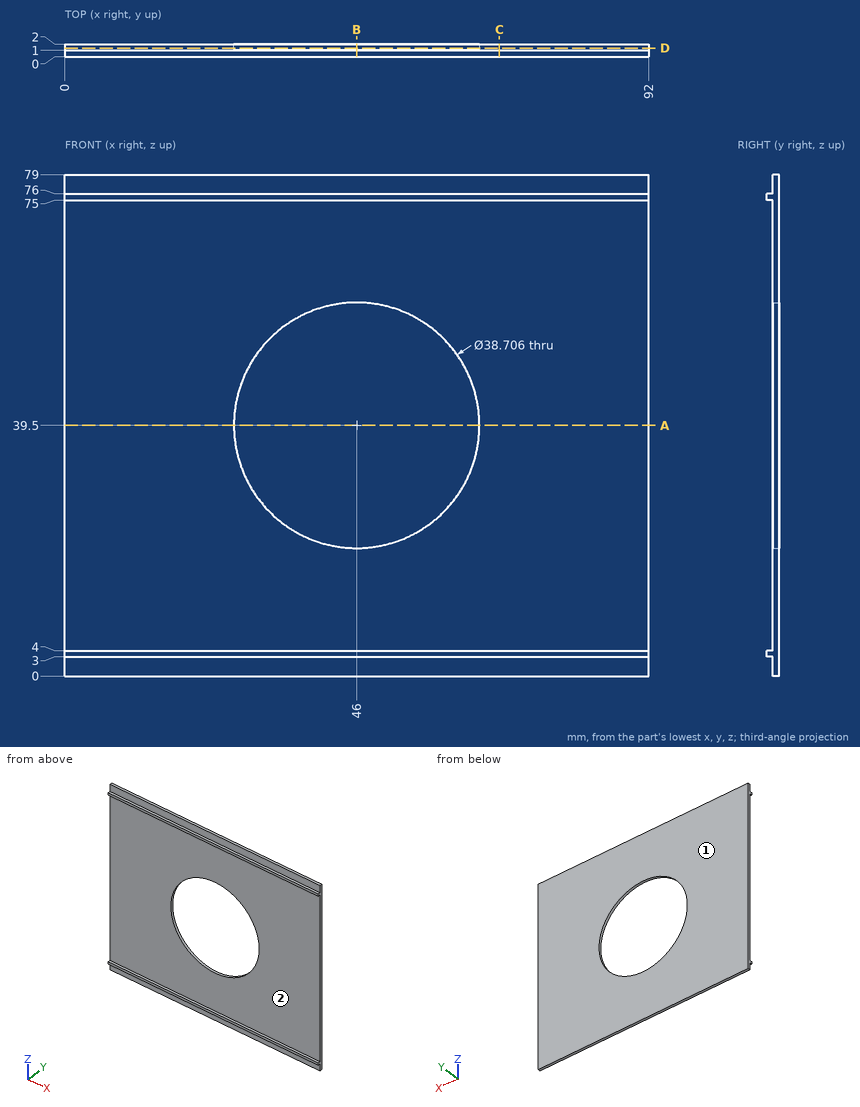
Could you check a few things on this drawing? It's one solid part, dimensions in mm from its lowest x, y, z. Coordinates: 2 decimals unless noted, no trailing zeros. Order: outer loops, then holes, each group sorted by start corner. A loop starts at its lowest first (then second) coordinate and runs counter-clockwise, first axis right, second up.
1) Will these pins go through, and if not, where does the flat tip stop? pin 1 (1.5 mm diameter, centred on x = 68.5, z = 78, fed in from -Y); pin 2 (0.8 mm diameter, centred on x = 43.5, y = 0.5, fed in from +Z); pin 3 (0.5 mm diameter, centred on x = 50.5, y = 0.5, fed in from -Z).
2) Imagine slicing it at C-C on x = 68.5. List the corners of the cut face in (y, z) for me.
3) Imagine slicing it at A-A on z = 39.5. List the corners of the cut face in (x, y) for me.
4) Imagine slicing it at B-B on x = 46. List the corners of the cut face in (y, z) for me.
5) I need wall thicknesses on line 1 (Z direction, x = 46, y = 1.55); line 2 (Z direction, x = 63, y = 0.7); line 3 (Y direction, x = 61.5, z = 52). Which ranges of each line are inside material? Lowest first, please.
6) Imagine slicing it at D-D on y = 1.35. List the corners of the cut face in (x, z) for me (1 decimal).
7) We'd pull the mould along Z, two halves only. Please class the marked faces 1 and 2: +Z half, -Z half, draft (parallel to the pull), parting line (faces both ways), or undercut.
Response values:
1. pin 1: stops at y = 1
1. pin 2: stops at z = 76
1. pin 3: stops at z = 3
2. outline: (0, 3) - (1, 3) - (1, 0) - (2, 0) - (2, 79) - (1, 79) - (1, 76) - (0, 76) - (0, 75) - (1, 75) - (1, 4) - (0, 4) - close
3. outline: (0, 1) - (26.65, 1) - (26.65, 2) - (0, 2) - close; (65.35, 1) - (92, 1) - (92, 2) - (65.35, 2) - close
4. outline: (0, 3) - (1, 3) - (1, 0) - (2, 0) - (2, 20.15) - (1, 20.15) - (1, 4) - (0, 4) - close; (0, 75) - (1, 75) - (1, 58.85) - (2, 58.85) - (2, 79) - (1, 79) - (1, 76) - (0, 76) - close
5. line 1: z = 0 to 20.15, 58.85 to 79
5. line 2: z = 3 to 4, 75 to 76
5. line 3: y = 1 to 2
6. outline: (0, 0) - (92, 0) - (92, 79) - (0, 79) - close; hole circle Ø38.7 at (46, 39.5)
7. face 1: draft
7. face 2: undercut
